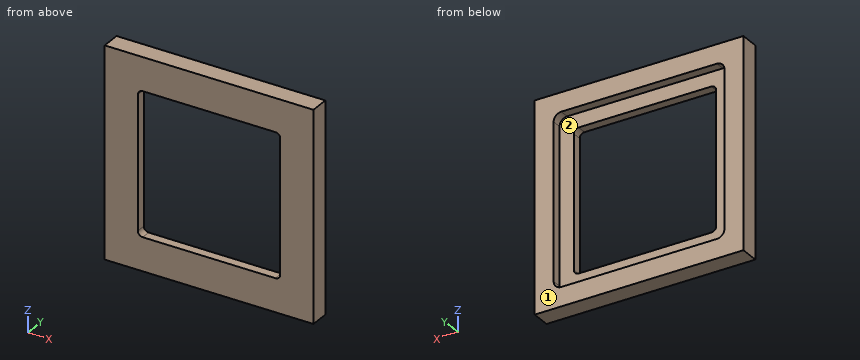
from build123d import *

# Parameters (mm, degrees)
SKETCH1_W           = 44
SKETCH1_H           = 44
SKETCH1_W_2         = 36
SKETCH1_H_2         = 36
BOSS_EXTRUDE1_DEPTH = 2
FILLET1_R           = 1.6
SKETCH2_W           = 44
SKETCH2_H           = 44
SKETCH2_W_2         = 30
SKETCH2_H_2         = 30
BOSS_EXTRUDE2_DEPTH = 2
FILLET2_R           = 1


with BuildPart() as part:
    # Sketch1 → Boss-Extrude1 (new body)
    with BuildSketch(Plane(origin=(0, 0, 0), x_dir=(1, 0, 0), z_dir=(0, 1, 0))):
        Rectangle(SKETCH1_W, SKETCH1_H)
        Rectangle(SKETCH1_W_2, SKETCH1_H_2, mode=Mode.SUBTRACT)
    extrude(amount=BOSS_EXTRUDE1_DEPTH)

    # Fillet1
    fillet1_edges = [part.edges().sort_by_distance(p)[0] for p in [
        (18, 1, -18),
        (-18, 1, -18),
        (-18, 1, 18),
        (18, 1, 18),
    ]]
    fillet(fillet1_edges, radius=FILLET1_R)

    # Sketch2 → Boss-Extrude2 (add)
    with BuildSketch(Plane.XZ):
        Rectangle(SKETCH2_W, SKETCH2_H)
        Rectangle(SKETCH2_W_2, SKETCH2_H_2, mode=Mode.SUBTRACT)
    extrude(amount=BOSS_EXTRUDE2_DEPTH)

    # Fillet2
    fillet2_edges = [part.edges().sort_by_distance(p)[0] for p in [
        (15, -1, 15),
        (-15, -1, 15),
        (-15, -1, -15),
        (15, -1, -15),
    ]]
    fillet(fillet2_edges, radius=FILLET2_R)


solid = part.part
Here's how the part is built. I have some questions about the finished solid (model axes, mm). Face numbers are marked on the shaded views. Coordinates: 2 decimals unless noted, no trailing zeros. Loops run counter-clockwise (first coordinate to the right, second up) from the corner with the lowest first, then second, coordinate; pieces in that order, holes last. Notation, with made-up numbers: (73.5, -5) -> (128.5, -5) arc R12 ccw to (128.5, 0) -> close; hole circle Ø7 at (-40, 36). An arc over 180 degrees is marked (long way). Use one line per item in the form item = value. Start each with the question number.
(1) If we section it at A-A (y = 1.1): Please give me the cut outline in (x, z), then the cut area to 3 significant figures.
(2) Please list where these lines run through material, in increasing order: line 1 along Z through (x, y) = (10, 1.8); line 2 along X through (y, z) = (-1.45, -10).
(3) If we section it at B-B (z = 4.5): Please give me the cut outline in (x, y), then the cut area to 3 significant figures.
(4) If we section it at C-C (x = -3.5): Please give me the cut outline in (y, z).
(5) If we section it at D-D (y = -1.1): Please give me the cut outline in (x, z).
(6) We'd pull the mould along Z, two halves only. Please class the marked faces 1 and 2: pulls with the +Z half, pulls with the -Z half, needs draft (parallel to the pull), parting line crosses it, or undercut.
Verdict:
q1.outline = (-22, -22) -> (22, -22) -> (22, 22) -> (-22, 22) -> close; hole (-18, -16.4) arc R1.6 ccw to (-16.4, -18) -> (16.4, -18) arc R1.6 ccw to (18, -16.4) -> (18, 16.4) arc R1.6 ccw to (16.4, 18) -> (-16.4, 18) arc R1.6 ccw to (-18, 16.4) -> close
q1.area = 642 mm²
q2.line_1 = -22 to -18, 18 to 22
q2.line_2 = -22 to -15, 15 to 22
q3.outline = (-22, -2) -> (-15, -2) -> (-15, 0) -> (-18, 0) -> (-18, 2) -> (-22, 2) -> close; (15, -2) -> (22, -2) -> (22, 2) -> (18, 2) -> (18, 0) -> (15, 0) -> close
q3.area = 44.0 mm²
q4.outline = (-2, -22) -> (2, -22) -> (2, -18) -> (0, -18) -> (0, -15) -> (-2, -15) -> close; (-2, 15) -> (0, 15) -> (0, 18) -> (2, 18) -> (2, 22) -> (-2, 22) -> close
q5.outline = (-22, -22) -> (22, -22) -> (22, 22) -> (-22, 22) -> close; hole (-15, -14) arc R1 ccw to (-14, -15) -> (14, -15) arc R1 ccw to (15, -14) -> (15, 14) arc R1 ccw to (14, 15) -> (-14, 15) arc R1 ccw to (-15, 14) -> close
q6.face_1 = needs draft
q6.face_2 = undercut
